The model under review builds one solid part; all positions refer to its coordinate system, in mm. Coordinates: 2 decimals unless noted, no trailing zeros. Loops run counter-clockwise (first coordinate to the right, second up) from the corner with the lowest first, then second, coordinate; pieces in that order, holes last. Notation, with made-up numbers: (42.5, 4) - (91.5, 4) arc R19 cw to (91.5, 18) - close; hole circle Ø10 at (1.25, 5.25). An arc over 180 degrees is marked (long way). Use a Markdown table: item, result. Add a question column.
1) To check wall thickness, follow L1, parallel to Z at x = 9, y = 1.7; L2, parallel to Z at x = 5, y = 0.6; L3, parallel to Z at x = 71.5, y = 1.7. State the ranges of each line that lie inside material, in increasing order. Write a range as [from, to].
2) Clearance check with flat-ended pins moving along their axes: pin 1 (1.1 mm diameter, centred on x = 73, y = 1, fed in from +Z); pin 2 (0.7 mm diameter, centred on y = 1, z = 92, fed in from +X); pin 3 (1.1 mm diameter, centred on y = 0.5, z = -27, fed in from -X); pin 4 (1 mm diameter, centred on x = 39.5, z = 32.5, fed in from -Y). State where each tip first meets the part, or that it passes through.
3) Add section A-A, the plane x = 18.5. Give the boundary of the cut face in (y, z), and give its area (3 significant figures).
4) Add section D-D, the plane y = 1.7. Give the number of separate pieces and of enclosed holes in the cut face, and give its area (3 significant figures).
5) Add section C-C, the plane x = -37. Give the boundary of the cut face in (y, z).
6) Add section B-B, the plane z = -15.5. Give the boundary of the cut face in (x, y).
```python
from build123d import *

# Parameters (mm, degrees)
SKETCH1_R           = 10
SKETCH1_R_2         = 15
BOSS_EXTRUDE1_DEPTH = 2.2


with BuildPart() as part:
    # Sketch1 → Boss-Extrude1 (new body)
    with BuildSketch(Plane(origin=(0, 0, 0), x_dir=(1, 0, 0), z_dir=(0, 1, 0))):
        with BuildLine():
            Line((28.996705531, 1.904265459), (33.969810226, 6.877370153))
            Line((33.969810226, 6.877370153), (31.141383101, 9.705797278))
            Line((31.141383101, 9.705797278), (31.141383101, 44.705797278))
            ThreePointArc((31.141383101, 44.705797278), (26.747984819, 55.312398995), (16.141383101, 59.705797278))
            Line((16.141383101, 59.705797278), (9.99459577, 59.705797278))
            ThreePointArc((9.99459577, 59.705797278), (-0.612005948, 55.312398995), (-5.00540423, 44.705797278))
            Line((-5.00540423, 44.705797278), (-5.00540423, 9.705797278))
            Line((-5.00540423, 9.705797278), (-30.56504267, -15.853841163))
            Line((-30.56504267, -15.853841163), (-65.56504267, -15.853841163))
            ThreePointArc((-65.56504267, -15.853841163), (-76.171644388, -20.247239445), (-80.56504267, -30.853841163))
            Line((-80.56504267, -30.853841163), (-80.56504267, -37.000628494))
            ThreePointArc((-80.56504267, -37.000628494), (-76.171644388, -47.607230212), (-65.56504267, -52.000628494))
            Line((-65.56504267, -52.000628494), (-33.289675478, -52.000628494))
            Line((-33.289675478, -52.000628494), (-30.843341676, -49.554294692))
            Line((-30.843341676, -49.554294692), (-28.773918492, -51.623717877))
            ThreePointArc((-28.773918492, -51.623717877), (-26.652598148, -52.502397534), (-24.531277804, -51.623717877))
            Line((-24.531277804, -51.623717877), (-22.763510851, -49.855950924))
            Line((-22.763510851, -49.855950924), (-21.349297289, -48.441737362))
            Line((-21.349297289, -48.441737362), (-14.985336258, -54.805698393))
            Line((-14.985336258, -54.805698393), (-13.571122696, -53.39148483))
            Line((-13.571122696, -53.39148483), (-6.396260567, -60.566346959))
            Line((-6.396260567, -60.566346959), (-7.810474129, -61.980560522))
            Line((-7.810474129, -61.980560522), (-1.446513098, -68.344521553))
            Line((-1.446513098, -68.344521553), (-2.860726661, -69.758735115))
            Line((-2.860726661, -69.758735115), (-4.628493614, -71.526502068))
            ThreePointArc((-4.628493614, -71.526502068), (-5.50717327, -73.647822411), (-4.628493614, -75.769142755))
            Line((-4.628493614, -75.769142755), (-2.559070429, -77.83856594))
            Line((-2.559070429, -77.83856594), (-5.00540423, -80.284899741))
            Line((-5.00540423, -80.284899741), (-5.00540423, -112.560266934))
            ThreePointArc((-5.00540423, -112.560266934), (-0.612005948, -123.166868652), (9.99459577, -127.560266934))
            Line((9.99459577, -127.560266934), (16.141383101, -127.560266934))
            ThreePointArc((16.141383101, -127.560266934), (26.747984819, -123.166868652), (31.141383101, -112.560266934))
            Line((31.141383101, -112.560266934), (31.141383101, -77.560266934))
            Line((31.141383101, -77.560266934), (33.969810226, -74.731839809))
            Line((33.969810226, -74.731839809), (28.996705531, -69.758735115))
            Line((28.996705531, -69.758735115), (27.582491969, -68.344521553))
            Line((27.582491969, -68.344521553), (33.946453, -61.980560522))
            Line((33.946453, -61.980560522), (32.532239437, -60.566346959))
            Line((32.532239437, -60.566346959), (39.707101567, -53.39148483))
            Line((39.707101567, -53.39148483), (41.121315129, -54.805698393))
            Line((41.121315129, -54.805698393), (47.48527616, -48.441737362))
            Line((47.48527616, -48.441737362), (48.899489722, -49.855950924))
            Line((48.899489722, -49.855950924), (53.872594416, -54.829055619))
            Line((53.872594416, -54.829055619), (56.701021541, -52.000628494))
            Line((56.701021541, -52.000628494), (91.701021541, -52.000628494))
            ThreePointArc((91.701021541, -52.000628494), (102.307623259, -47.607230212), (106.701021541, -37.000628494))
            Line((106.701021541, -37.000628494), (106.701021541, -30.853841163))
            ThreePointArc((106.701021541, -30.853841163), (102.307623259, -20.247239445), (91.701021541, -15.853841163))
            Line((91.701021541, -15.853841163), (56.701021541, -15.853841163))
            Line((56.701021541, -15.853841163), (53.872594416, -13.025414038))
            Line((53.872594416, -13.025414038), (48.899489722, -17.998518732))
            Line((48.899489722, -17.998518732), (47.48527616, -19.412732294))
            Line((47.48527616, -19.412732294), (41.121315129, -13.048771264))
            Line((41.121315129, -13.048771264), (39.707101567, -14.462984826))
            Line((39.707101567, -14.462984826), (32.532239437, -7.288122697))
            Line((32.532239437, -7.288122697), (33.946453, -5.873909135))
            Line((33.946453, -5.873909135), (27.582491969, 0.490051896))
            Line((27.582491969, 0.490051896), (28.996705531, 1.904265459))
        make_face()
        with Locations(Location((-55.56504267, -33.927234828, 0), (0, 0, 270))):
            Circle(SKETCH1_R, mode=Mode.SUBTRACT)
        with Locations(Location((13.067989435, -102.560266934, 0), (0, 0, 270))):
            Circle(SKETCH1_R, mode=Mode.SUBTRACT)
        with Locations(Location((13.067989435, -33.927234828, 0), (0, 0, 270))):
            Circle(SKETCH1_R_2, mode=Mode.SUBTRACT)
        with Locations(Location((81.701021541, -33.927234828, 0), (0, 0, 270))):
            Circle(SKETCH1_R, mode=Mode.SUBTRACT)
        with Locations(Location((13.067989435, 34.705797278, 0), (0, 0, 270))):
            Circle(SKETCH1_R, mode=Mode.SUBTRACT)
    extrude(amount=BOSS_EXTRUDE1_DEPTH)


solid = part.part
```
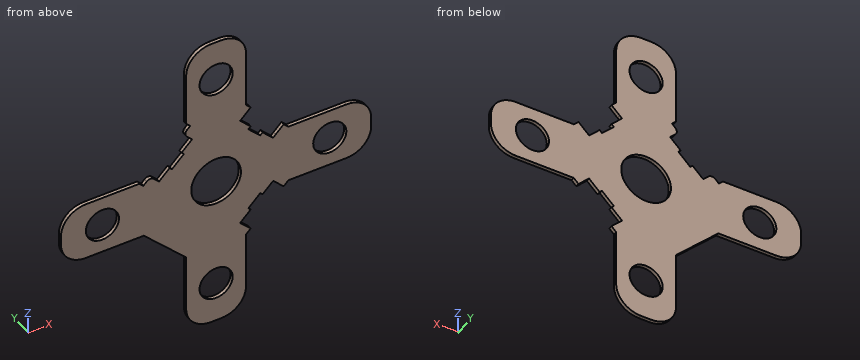
From the geometry:
| question | item | result |
|---|---|---|
| 1 | L1 | z = [-59.67, -43.84], [-25.57, 19.49], [48.37, 93.43], [111.7, 127.53] |
| 1 | L2 | z = [-58.85, -40.61], [-28.8, 21.28], [46.57, 96.65], [108.47, 126.7] |
| 1 | L3 | z = [15.85, 52] |
| 2 | pin 1 | stops at z = 52 |
| 2 | pin 2 | stops at x = 31.14 |
| 2 | pin 3 | stops at x = -5.01 |
| 2 | pin 4 | stops at y = 0 |
| 3 | outline | (0, -59.52) - (2.2, -59.52) - (2.2, -43.1) - (0, -43.1) - close; (0, -26.31) - (2.2, -26.31) - (2.2, 19.95) - (0, 19.95) - close; (0, 47.91) - (2.2, 47.91) - (2.2, 94.16) - (0, 94.16) - close; (0, 110.96) - (2.2, 110.96) - (2.2, 127.37) - (0, 127.37) - close |
| 3 | area | 276 mm^2 |
| 4 | separate pieces | 1 |
| 4 | enclosed holes | 5 |
| 4 | area | 10,300 mm^2 |
| 5 | outline | (0, 15.85) - (2.2, 15.85) - (2.2, 52) - (0, 52) - close |
| 6 | outline | (-5.01, 0) - (31.14, 0) - (31.14, 2.2) - (-5.01, 2.2) - close |
